Could you check a few things on this drawing? It's one solid part, dimensions in mm from its lowest x, y, z. A direction names the side the tool comes from. Round coordinates to 2 decimals unless told otherwise and drop trailing zeros. Loops run counter-clockwise (first coordinate to the right, second up) from the corner with the lowest first, then second, coordinate; pieces in that order, holes last. Notation, with made-up numbers: (44.5, 80.5) -> (88.5, 80.5) arc R20 cw to (88.5, 85.5) -> close; hole circle Ø10 at (82.25, -10.75). An arc over 180 degrees is marked (long way). Put each result on its own line as item: value. Start each with the question number.
1. Imagine slicing it at D-D, the plane z = 74. Please give me the cut outline in (x, y), and give its area (3 significant figures).
2. Which directions (+Z, -Z, +X, -X, +Y, -Y) give clear straight access to the entire face, cutting with the end or side of a thin tool? Please do the marked faces 1 and 2.
3. I'm going to push flat-ended pins straight in: P1, Ø6, axis at y = 73, z = 51.5, coming from the +X side; P2, Ø1.5, axis at x = 23.5, z = 64, coming from the -Y side; P3, Ø4, axis at y = 36.5, z = 48, coming from the -X side; P4, Ø6, axis at x = 10, y = 81, coming from the +Z side. Where does each tip first touch, or does it pass through?
4. If we mould it in two halves opening along Y, with no side actions, what happens to the marked faces 3, 4 and 5? For each: pulls with the +Y half, pulls with the -Y half, needs draft (parallel to the pull), parting line crosses it, or undercut.
5. Imagine slicing it at C-C, the plane z = 148.5. Please give me the cut outline in (x, y), and give its area (3 significant figures).
6. I need wall thicknesses on line 1 (Y direction, x = 45, z = 152); line 2 (Z direction, x = 45, y = 45); line 3 (Z direction, x = 55, y = 12). Which ranges of each line are inside material? Lowest first, please. Write a range as [from, to].
7. Imagine slicing it at B-B, the plane y = 45. Please give me the cut outline in (x, z).
8. Imagine slicing it at A-A, the plane x = 45. Please give me the cut outline in (y, z).
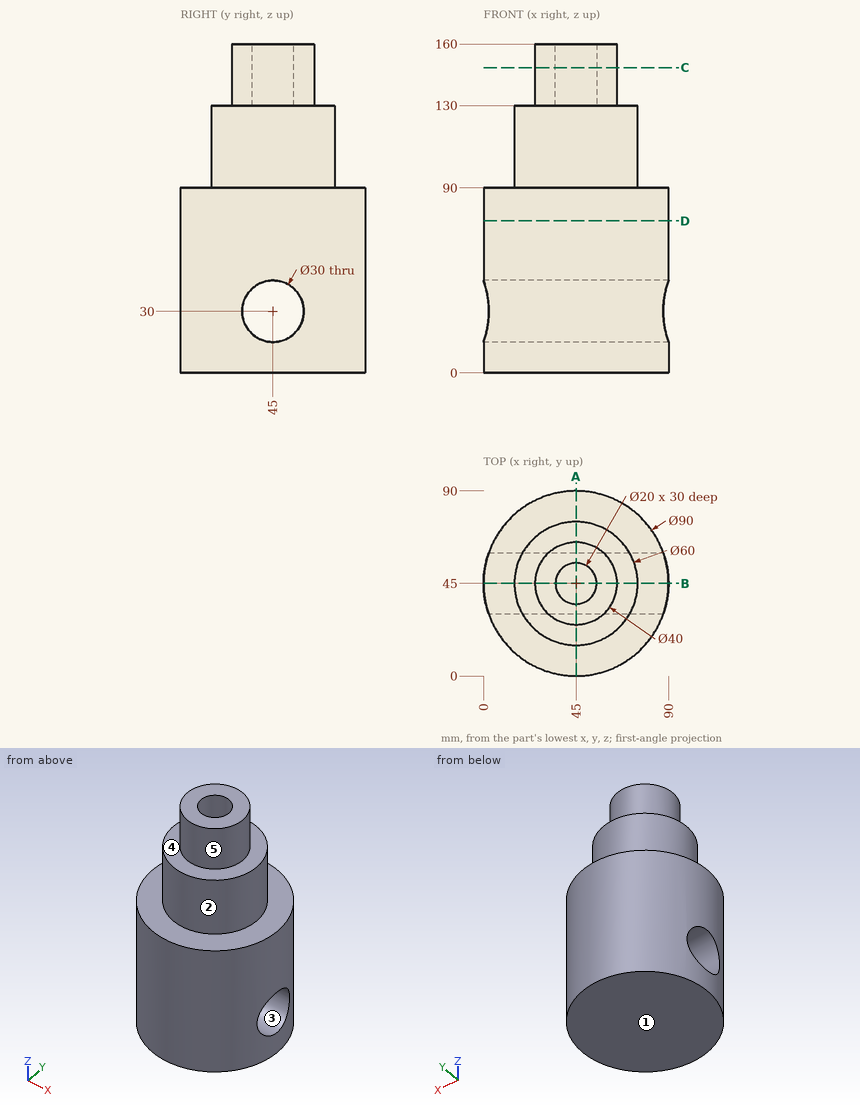
Entries:
1. outline: circle Ø90 at (45, 45)
1. area: 6,360 mm^2
2. face 1: -Z, +X, -X, +Y, -Y
2. face 2: +Z
3. P1: x = 82.42
3. P2: y = 5.07
3. P3: x = 0.47
3. P4: through
4. face 3: undercut
4. face 4: needs draft
4. face 5: parting line crosses it
5. outline: circle Ø40 at (45, 45); hole circle Ø20 at (45, 45)
5. area: 942 mm^2
6. line 1: [25, 35], [55, 65]
6. line 2: [0, 15], [45, 130]
6. line 3: [0, 90]
7. outline: (0, 0) -> (90, 0) -> (90, 15) -> (0, 15) -> close; (0, 45) -> (90, 45) -> (90, 90) -> (75, 90) -> (75, 130) -> (65, 130) -> (65, 160) -> (55, 160) -> (55, 130) -> (35, 130) -> (35, 160) -> (25, 160) -> (25, 130) -> (15, 130) -> (15, 90) -> (0, 90) -> close
8. outline: (0, 0) -> (90, 0) -> (90, 90) -> (75, 90) -> (75, 130) -> (65, 130) -> (65, 160) -> (55, 160) -> (55, 130) -> (35, 130) -> (35, 160) -> (25, 160) -> (25, 130) -> (15, 130) -> (15, 90) -> (0, 90) -> close; hole circle Ø30 at (45, 30)
